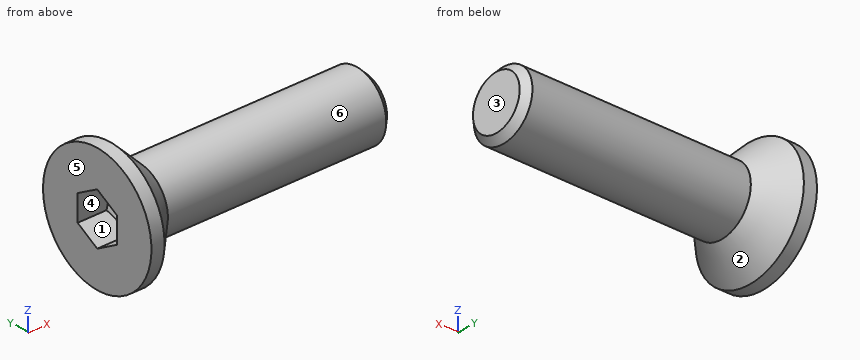
Autodesk Inventor part; units mm, degrees
ref_plane "Work Plane1" through (104.775, 0, 0) normal (0, 0, -1) x (1, 0, 0)
ref_plane "YZ Plane" through (0, 0, 0) normal (1, 0, 0) x (0, 1, 0)
ref_plane "XZ Plane" through (0, 0, 0) normal (0, 1, 0) x (-1, 0, 0)
sketch "Sketch1" plane through (0, 0, 0) normal (0, 0, 1) x (1, 0, 0)
  line L0 (12, 0) -> (12, 1.5)
  line L1 (12, 1.5) -> (4, 1.5)
  line L2 (4, 1.5) -> (3.6933, 1.5)
  line L3 (0, 2.77) -> (0, 1.1547)
  line L4 (0, 1.1547) -> (1.3, 1.1547)
  line L5 (1.3, 1.1547) -> (1.9667, 0)
  line L6 (1.9667, 0) -> (12, 0)
  line L7 (0, 2.77) -> (0.59, 2.77)
  line L8 (0.59, 2.77) -> (1.86, 1.5)
  line L9 (3.6933, 1.5) -> (1.86, 1.5)
  line L10 (4, 1.5) -> (1.86, 1.5) construction
  line L11 (1.86, 1.5) -> (1.86, 1.5)
  line L12 (-2.4, 0) -> (14.4, 0)
  line L13 (0, -0.554) -> (0, 3.324)
  dimension "d0" = 12
  dimension "d1" = 8
  dimension "d2" = 1.3
  dimension "d3" = 3
  dimension "d6" = 1.86
  dimension "d7" = 45
  dimension "d8" = 2.3094
  dimension "d9" = 60
  dimension "d10" = 5.54
  dimension "d11" = 3
  dimension "d12" = 0.3067
revolve "Body" add sketch "Sketch1" angle 360 about axis through (1.9667, 0, 0) along (1, 0, 0) contours L6 L5 L4 L3 L7 L8 L9 L2 L1 L0
sketch "Sketch2" plane through (0, 0, 0) normal (-1, 0, 0) x (0, 0, 1)
  circle A0 centre (0, 0) radius 1.1547
  line L0 (0, -3.878) -> (0, 3.878)
  line L1 (-3.878, 0) -> (3.878, 0)
  line L2 (1.1547, 0) -> (0.5774, -1)
  line L3 (0.5774, -1) -> (-0.5774, -1)
  line L4 (-0.5774, -1) -> (-1.1547, 0)
  line L5 (-1.1547, 0) -> (-0.5774, 1)
  line L6 (-0.5774, 1) -> (0.5774, 1)
  line L7 (0.5774, 1) -> (1.1547, 0)
  point P0 (0, 1.1547)
extrude "Slot" add sketch "Sketch2" against normal up to next contours L7 A0 | A0 L2 | L6 L0 A0 | A0 L0 L3 | L0 L6 A0 | A0 L3 L0 | L4 A0 | A0 L5
thread "Thread"
chamfer "Chamfer1" distance 0.3067 distance2 0.3067 1 edges at (12, -1.5, 0) measured on face at (12, -0.3743, -0.3316)
ref_plane "Work Plane1" through (104.775, 0, 0) normal (0, 0, -1) x (1, 0, 0)
equation "\"d0\" = NLG"
equation "\"d1\" = GEL"
equation "\"d2\" = INTI"
equation "\"d3\" = GD"
equation "\"d6\" = KOH"
equation "\"d7\" = 0.5 * SEWI"
equation "\"d8\" = 1.1547 * SW"
equation "\"d10\" = KOD"
equation "\"d11\" = BDM"
equation "\"d12\" = GAL"
equation "\"d15\" = GEL"
equation "\"d17\" = -0.5 * SPD + 0.5 * GD"
equation "\"d18\" = GUL"
equation "\"NLG\" = 12"
equation "\"INTI\" = 1.3"
equation "\"GEL\" = 8"
equation "\"GAL\" = 0.61345 * PTC"
equation "\"KOH\" = 1.86"
equation "\"KOD\" = 5.54"
equation "\"GUL\" = 0.61345 * PTC"
equation "\"SPD\" = NND - 1.2269 * PTC"
equation "\"BDM\" = NND"
equation "\"GD\" = NND"
equation "\"SEWI\" = 90deg"
equation "\"SW\" = 2"
equation "\"TOA\" = 30deg"
equation "\"GD1\" = THREADDIA - 1.2269 * PTC"
equation "\"EPV\" = 3.36"
equation "\"THREADDIA\" = 3"
equation "\"PTC\" = 0.5"
equation "\"NND\" = 3"
equation "\"E0\" = 2.31"
equation "\"THREADDESC\" = 1.2345"
properties part number "M3 x  12 - Socket Csk Screw (A2)" material "Stainless Steel"
The model under review builds one solid part; all positions refer to its coordinate system, in mm. Face numbers are marked on the shaded views. A direction names the side the tool comes from. Round coordinates to 2 decimals unless told otherwise and drop trailing zeros. Loops run counter-clockwise (first coordinate to the right, second up) from the corner with the lowest first, then second, coordinate; pieces in that order, holes last. Notation, with made-up numbers: (76.25, 41.25) -> (84.25, 41.25) arc R28 cw to (84.25, 64.25) -> close; hole circle Ø3 at (24, 3). An arc over 180 degrees is marked (long way). Return JSON: item names as keys, results as strings.
(1) For pin 1 (1 mm diameter, centred on x = 9.5, y = 0.5, fed in from -Z), flat-tipped, find the tip position at first contact; note if it passes through.
Solved:
{"pin 1": "z = -1.5"}
(2) The part is to be moulded in two halves that separate along Y. For the marked faces 1, 2, 3 and 4, say which applies: released by +Y, released by -Y, zero draft, split by the parting line, or undercut.
Solved:
{"face 1": "undercut", "face 2": "split by the parting line", "face 3": "zero draft", "face 4": "undercut"}
(3) Add section A-A on x = 3.25. Write out the cut boundary in (y, z), plus the area to 3 significant figures.
Solved:
{"outline": "circle Ø3 at (0, 0)", "area": "7.07 mm2"}
(4) For the marked faces 5 and 6, list the 3-axis set-ups (+Z, -Z, +X, -X, +Y, -Y) from which the entire face can be reached by the end or side of a thin tool; tool diameter is ignored.
Solved:
{"face 5": "+Z, -Z, -X, +Y, -Y", "face 6": "+X"}
(5) For line 1 (Z direction, x = 9.25, y = -0.05); line 2 (Z direction, x = 1, y = 0.95); line 3 (X direction, y = 0.35, z = 2.25), list the stretches that pass through material, from the lowest coordinate up.
Solved:
{"line 1": "-1.5 to 1.5", "line 2": "-2.16 to -0.61, 0.61 to 2.16", "line 3": "0 to 1.08"}
